```python
from build123d import *

# Parameters (mm, degrees)
SKETCH1_R           = 2.15
BOSS_EXTRUDE1_DEPTH = 3.78


with BuildPart() as part:
    # Sketch1 → Boss-Extrude1 (new body)
    with BuildSketch(Plane(origin=(0, 0, 0), x_dir=(1, 0, 0), z_dir=(0, 1, 0))):
        Polygon((4.578387635, 0), (2.289193817, 3.965), (-2.289193817, 3.965), (-4.578387635, 0), (-2.289193817, -3.965), (2.289193817, -3.965), align=None)
        with Locations(Location((0, 0, 0), (0, 0, 270))):
            Circle(SKETCH1_R, mode=Mode.SUBTRACT)
    extrude(amount=BOSS_EXTRUDE1_DEPTH)

    # Sketch2 → Cut-Revolve1 (revolve, cut)
    with BuildSketch(Plane(origin=(0, 0, 0), x_dir=(0, 0, -1), z_dir=(1, 0, 0)), mode=Mode.PRIVATE) as cut_revolve1_sk:
        Polygon((3.008379415, 4.316956257), (7.760790511, 0.730297909), (8.861229965, 2.9800107), align=None)
    revolve(cut_revolve1_sk.sketch.rotate(Axis((0, 0, 0), (0, 1, 0)), 329.999999889), axis=Axis((0, 0, 0), (0, 1, 0)), mode=Mode.SUBTRACT)


solid = part.part
```
CAD build for the part. Positions are in the model's coordinates, mm. Round coordinates to 2 decimals unless told otherwise and drop trailing zeros. Write each loop counter-clockwise with the first axis right and the second up, starting at its lowest first coordinate (ties: lowest second). Pieces come first, ordered by that corner, then holes.
Item 1: Band-saw the part on A-A on y = 2.55. Write the cut outline in (x, z) (3 decimals), then the cut area to 3 significant figures.
Filled in:
outline: (-4.578, 0) - (-2.289, -3.965) - (2.289, -3.965) - (4.578, 0) - (2.289, 3.965) - (-2.289, 3.965) - close; hole circle Ø4.3 at (0, 0)
area: 39.9 mm2
Item 2: Drop flat-ended pins along their axis: pin 1 Ø1.5 at (y, z) = (3, 2.5) entering from -X; pin 2 Ø1 at (x, y) = (-3.5, 0.5) entering from +Z; pin 3 Ø1.5 at (y, z) = (2.5, -3) entering from -X. Give the stop position or say it passes through.
Filled in:
pin 1: stops at x = -3.57
pin 2: stops at z = 2.73
pin 3: stops at x = -3.28
Item 3: Mould opens along X. For faces 1 (the cylindrical face through (-1.308, 1.864, -1.706)), 2 (the flat face through (2, 3.78, 2)), 3 (the flat face through (3.42, 1.77, 2.01)) say: released by +X, released by -X, zero draft, split by the parting line, or undercut.
Filled in:
face 1: undercut
face 2: zero draft
face 3: released by +X
Item 4: Drill centre lines: L1, parallel to X at y = 2.25, z = -1.75; L2, parallel to Z at x = 1, y = 2.35 (3 decimals); L3, parallel to X at y = 1.1, z = -1.5. Where is each one in solid material? Low to high.
Filled in:
L1: x = -3.57 to -1.25, 1.25 to 3.57
L2: z = -3.965 to -1.903, 1.903 to 3.965
L3: x = -3.71 to -1.54, 1.54 to 3.71
Item 5: Band-saw the part on B-B on x = 0. Write the cut outline in (y, z) (3 decimals), then the cut area to 3 significant figures.
Filled in:
outline: (0, -3.965) - (3.595, -3.965) - (3.78, -3.72) - (3.78, -2.15) - (0, -2.15) - close; (0, 2.15) - (3.78, 2.15) - (3.78, 3.72) - (3.595, 3.965) - (0, 3.965) - close
area: 13.7 mm2
